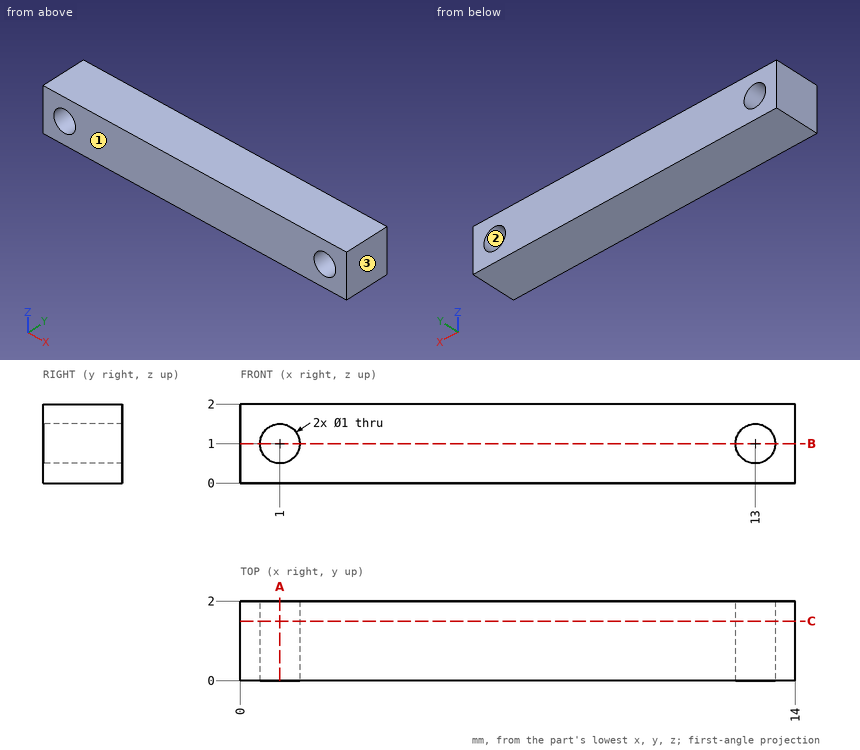
Check sheet for the drawn part. Datum: minimum x, y, z corner. Units: mm. Give positions to 0.01 mm unless a question says otherwise; leave off trailing zeros. Write each loop counter-clockwise with the first axis right and the second up, starting at its lowest first coordinate (ties: lowest second). Pieces come first, ordered by that corner, then holes. Notation, with made-up numbers: M -12.75,-4.75 L 36.25,-4.75 A21 cw 36.25,29.25 Z; hole C 80.5,-13 d5. An arc over 180 degrees is marked long. One line per question, with ' | ' between items.
1. Cross-section at A-A (x = 1). Enter the section's corners in (y, z).
Ans:
outline: M 0,0 L 2,0 L 2,0.5 L 0,0.5 Z; M 0,1.5 L 2,1.5 L 2,2 L 0,2 Z
2. Cross-section at B-B (z = 1). Enter the section's corners in (x, y).
Ans:
outline: M 0,0 L 0.5,0 L 0.5,2 L 0,2 Z; M 1.5,0 L 12.5,0 L 12.5,2 L 1.5,2 Z; M 13.5,0 L 14,0 L 14,2 L 13.5,2 Z
3. Scan lines: line 1 along Z through (x, y) = (13, 1.3); line 2 along X through (y, z) = (0.2, 0.75); line 3 along X through (y, z) = (1.45, 0.6). Record each from-to range of solid material in increasing order. Write a range as from..to.
Ans:
line 1: 0..0.5, 1.5..2 | line 2: 0..0.57, 1.43..12.57, 13.43..14 | line 3: 0..0.7, 1.3..12.7, 13.3..14
4. Cross-section at C-C (y = 1.5). Enter the section's corners in (x, z).
Ans:
outline: M 0,0 L 14,0 L 14,2 L 0,2 Z; hole C 1,1 d1; hole C 13,1 d1
5. Mould release check, pull along X, two halves, no side actions. Record for the marked faces 1, 2 and 3: released by +X, released by -X, zero draft, split by the parting line, or undercut.
Ans:
face 1: zero draft | face 2: undercut | face 3: released by +X
